from build123d import *

# Parameters (mm, degrees)
F4_T = -0.4


with BuildPart() as f3:
    # F0 (on Top) → F3 section 0
    with BuildSketch(Plane.XY):
        Polygon((12.7, 21.9970452561), (-12.7, 21.9970452561), (-25.4, 0), (-12.7, -21.9970452561), (12.7, -21.9970452561), (25.4, 0), align=None)
    # F2 (on offset) → F3 section 1
    with BuildSketch(Plane.XY.offset(12.7)):
        Polygon((-0.0081428164, 25.3999986948), (-22.001115534, 12.6929474615), (-21.9929727176, -12.7070512333), (0.0081428164, -25.3999986948), (22.001115534, -12.6929474615), (21.9929727176, 12.7070512333), align=None)
    loft()

    # F4
    f4_openings = [f3.faces().sort_by_distance(p)[0] for p in [
        (0, 0, 12.7),
    ]]
    offset(amount=F4_T, openings=f4_openings, kind=Kind.INTERSECTION)


solid = f3.part
Geometry check sheet. Reference: the model listing, model coordinates, mm. Round coordinates to 2 decimals unless told otherwise and drop trailing zeros. One line per question, with ' | ' between items. Start each with the question number.
1. Scan lines: line 1 (Y direction, x = -3, z = 6.75); line 2 (Y direction, x = -20.5, z = 2.5); line 3 (Z direction, x = -12, y = 17). Record each from-to range of solid material in increasing order. Write a range as [from, to].
2. Depth check by flat-ended pin: pin 1 (6 mm diameter, centred on y = 10.5, z = 6, fed in from -X); pin 2 (3 mm diameter, centred on y = 15, z = 6.5, fed in from -X); pin 3 (5 mm diameter, centred on x = -13.5, z = 3.5, fed in from -Y). Enter the tip coordinate at first touch or a pass-through.
3. Draft check along X on faces 1 (the face through (-20.3, -13.5, 12.7)), 2 (the face through (0, 0, 0.4)). Enter one of: released by +X, released by -X, zero draft, split by the parting line, or undercut.
Taken from the geometry:
1) line 1: [-21.25, -20.83], [22.51, 22.96] | line 2: [-6.9, -5.89], [7.68, 8.37] | line 3: [0, 0.4]
2) pin 1: x = -22.97 | pin 2: x = -16.59 | pin 3: y = -21.27
3) face 1: zero draft | face 2: undercut
